Design review of the part built by this model. Coordinates are the model's own, in mm. Round coordinates to 2 decimals unless told otherwise and drop trailing zeros. Loops run counter-clockwise (first coordinate to the right, second up) from the corner with the lowest first, then second, coordinate; pieces in that order, holes last. Notation, with made-up numbers: (-27, -36.75) -> (12, -36.75) arc R21 cw to (12, -17.75) -> close; hole circle Ø3 at (83, 42.25). An arc over 180 degrees is marked (long way). Use a Markdown table: item, result. Add a question column.
from build123d import *

# Parameters (mm, degrees)
BOSS_EXTRUDE1_DEPTH = 3
SKETCH2_R           = 1.5
SKETCH2_W           = 12
SKETCH2_H           = 3
SKETCH2_H_2         = 2.8
SKETCH2_W_2         = 20
CUT_EXTRUDE1_DEPTH  = 3
SKETCH4_R           = 1.6
CUT_EXTRUDE3_DEPTH  = 3
SKETCH5_R           = 1.5
SKETCH5_R_2         = 1.475
CUT_EXTRUDE4_DEPTH  = 3
SKETCH6_R           = 0.75
CUT_EXTRUDE5_DEPTH  = 3
CUT_EXTRUDE6_DEPTH  = 3


with BuildPart() as part:
    # Sketch1 → Boss-Extrude1 (new body)
    with BuildSketch(Plane(origin=(0, 0, 0), x_dir=(1, 0, 0), z_dir=(0, 1, 0))):
        with BuildLine():
            Line((100, -65), (-100, -65))
            ThreePointArc((-100, -65), (-107.071067812, -62.071067812), (-110, -55))
            Line((-110, -55), (-110, 55))
            ThreePointArc((-110, 55), (-107.071067812, 62.071067812), (-100, 65))
            Line((-100, 65), (100, 65))
            ThreePointArc((100, 65), (107.071067812, 62.071067812), (110, 55))
            Line((110, 55), (110, -55))
            ThreePointArc((110, -55), (107.071067812, -62.071067812), (100, -65))
        make_face()
    extrude(amount=BOSS_EXTRUDE1_DEPTH)

    # Sketch2 → Cut-Extrude1 (cut)
    with BuildSketch(Plane(origin=(0, 3, 0), x_dir=(1, 0, 0), z_dir=(0, 1, 0))):
        with Locations(Location((-85, 18.5, 0), (0, 0, 270))):
            Circle(SKETCH2_R)
        with Locations(Location((-48, 18.5, 0), (0, 0, 270))):
            Circle(SKETCH2_R)
        with Locations(Location((-85, -18.5, 0), (0, 0, 270))):
            Circle(SKETCH2_R)
        with Locations(Location((-48, -18.5, 0), (0, 0, 270))):
            Circle(SKETCH2_R)
        with Locations(Location((48, -18.5, 0), (0, 0, 90))):
            Circle(SKETCH2_R)
        with Locations(Location((85, -18.5, 0), (0, 0, 90))):
            Circle(SKETCH2_R)
        with Locations(Location((48, 18.5, 0), (0, 0, 90))):
            Circle(SKETCH2_R)
        with Locations(Location((85, 18.5, 0), (0, 0, 90))):
            Circle(SKETCH2_R)
        with Locations(Location((0, -57.5, 0), (0, 0, 270))):
            Circle(SKETCH2_R)
        with Locations(Location((0, 57.5, 0), (0, 0, 90))):
            Circle(SKETCH2_R)
        with Locations((64, -63.5)):
            Rectangle(SKETCH2_W, SKETCH2_H)
        with Locations((64, 63.5)):
            Rectangle(SKETCH2_W, SKETCH2_H)
        with Locations((-64, -63.5)):
            Rectangle(SKETCH2_W, SKETCH2_H)
        with Locations((-64, 63.6)):
            Rectangle(SKETCH2_W, SKETCH2_H_2)
        with Locations((-64, 41.7)):
            Rectangle(SKETCH2_W, SKETCH2_H)
        with Locations((64, 41.5)):
            Rectangle(SKETCH2_W, SKETCH2_H)
        with Locations((64, -41.5)):
            Rectangle(SKETCH2_W, SKETCH2_H)
        with Locations((-64, -41.5)):
            Rectangle(SKETCH2_W, SKETCH2_H)
        with Locations((29.820667629, -57.5)):
            Rectangle(SKETCH2_W_2, SKETCH2_H)
        with Locations((-29.820667629, -57.5)):
            Rectangle(SKETCH2_W_2, SKETCH2_H)
        with Locations((-29.820667629, 57.5)):
            Rectangle(SKETCH2_W_2, SKETCH2_H)
        with Locations((29.820667629, 57.5)):
            Rectangle(SKETCH2_W_2, SKETCH2_H)
    extrude(amount=-CUT_EXTRUDE1_DEPTH, mode=Mode.SUBTRACT)

    # Sketch4 → Cut-Extrude3 (cut)
    with BuildSketch(Plane(origin=(0, 3, 0), x_dir=(1, 0, 0), z_dir=(0, 1, 0))):
        with Locations(Location((26.468228909, -27.625, 0), (0, 0, 270))):
            Circle(SKETCH4_R)
        with Locations(Location((45.718228909, 27.625, 0), (0, 0, 270))):
            Circle(SKETCH4_R)
    extrude(amount=-CUT_EXTRUDE3_DEPTH, mode=Mode.SUBTRACT)

    # Sketch5 → Cut-Extrude4 (cut)
    with BuildSketch(Plane.XZ):
        with Locations(Location((-27.638314588, -20, 0), (0, 0, 270))):
            Circle(SKETCH5_R)
        with Locations(Location((-8.638314588, 20, 0), (0, 0, 270))):
            Circle(SKETCH5_R)
        with Locations(Location((22.163922177, 15.1, 0), (0, 0, 270))):
            Circle(SKETCH5_R_2)
        with Locations(Location((5.913922177, -15.1, 0), (0, 0, 270))):
            Circle(SKETCH5_R_2)
    extrude(amount=-CUT_EXTRUDE4_DEPTH, mode=Mode.SUBTRACT)

    # Sketch6 → Cut-Extrude5 (cut)
    with BuildSketch(Plane(origin=(0, 3, 0), x_dir=(1, 0, 0), z_dir=(0, 1, 0))):
        with Locations(Location((101.22716255, -21.591786593, 0), (0, 0, 270))):
            Circle(SKETCH6_R)
        with Locations(Location((97.22716255, 20.608213407, 0), (0, 0, 270))):
            Circle(SKETCH6_R)
    extrude(amount=-CUT_EXTRUDE5_DEPTH, mode=Mode.SUBTRACT)

    # Sketch7 → Cut-Extrude6 (cut)
    with BuildSketch(Plane(origin=(0, 3, 0), x_dir=(1, 0, 0), z_dir=(0, 1, 0))):
        with BuildLine():
            Line((-25, -44.5), (25, -44.5))
            ThreePointArc((25, -44.5), (28.5, -48), (25, -51.5))
            Line((25, -51.5), (-25, -51.5))
            ThreePointArc((-25, -51.5), (-28.5, -48), (-25, -44.5))
        make_face()
        with BuildLine():
            Line((-25, 51.5), (25, 51.5))
            ThreePointArc((25, 51.5), (28.5, 48), (25, 44.5))
            Line((25, 44.5), (-25, 44.5))
            ThreePointArc((-25, 44.5), (-28.5, 48), (-25, 51.5))
        make_face()
    extrude(amount=-CUT_EXTRUDE6_DEPTH, mode=Mode.SUBTRACT)


solid = part.part
1. Consider section B-B on y = 2.2. Give the number of separate pieces and of enclosed holes in the cut face, plus the area to 3 significant figures.
2. Insertion check: P1, Ø2.5, axis at x = -85, z = 18.5, coming from the -Y side; P2, Ø1.5, axis at x = 63.5, y = 2, coming from the +Z side. Each pin has a flat end and moves straight along its axis. Give the tip position at first contact, or say it passes through.
3. Consider section A-A on z = 48. State the section outline as (x, y) points, plus the area to 3 significant figures.
4. To check wall thickness, follow probe 1 along Z at (x, y) = (-24, 1.4); probe 2 along Z at (x, y) = (-14, 0.2); probe 3 along Z at (x, y) = (32, 0.35). State the ranges of each line that lie inside material, in increasing order. Write a range as from..to.
Verdict:
| question | item | result |
|---|---|---|
| 1 | separate pieces | 1 |
| 1 | enclosed holes | 28 |
| 1 | area | 27,100 mm² |
| 2 | P1 | passes through |
| 2 | P2 | stops at z = 62 |
| 3 | outline | (-110, 0) -> (-28.5, 0) -> (-28.5, 3) -> (-110, 3) -> close; (28.5, 0) -> (110, 0) -> (110, 3) -> (28.5, 3) -> close |
| 3 | area | 489 mm² |
| 4 | probe 1 | z = -65..-59, -56..-51.5, -44.5..44.5, 51.5..56, 59..65 |
| 4 | probe 2 | z = -65..-51.5, -44.5..44.5, 51.5..65 |
| 4 | probe 3 | z = -65..-59, -56..56, 59..65 |
